The model under review builds one solid part; all positions refer to its coordinate system, in mm. Face numbers are marked on the shaded views. A direction names the side the tool comes from. Round coordinates to 2 decimals unless told otherwise and drop trailing zeros. Return JSON: item names as keys, results as strings.
from build123d import *

# Parameters (mm, degrees)
SKETCH_4_W             = 1
SKETCH_4_H             = 1.2
CUT_EXTRUDE_1_DEPTH    = 50
PATTERN_LINEAR_1_COUNT = 19
PATTERN_LINEAR_1_PITCH = 0.7


with BuildPart() as part:
    # 草图3 → Revolve 915 (revolve)
    with BuildSketch(Plane.XY, mode=Mode.PRIVATE) as revolve_915_sk:
        with BuildLine():
            Line((0, 0), (16.4, 0))
            Line((16.4, 0), (16.4, 2))
            Line((16.4, 2), (3.8, 2))
            Line((3.8, 2), (3.532, 1.732))
            Line((3.532, 1.732), (3.018, 1.732))
            ThreePointArc((3.018, 1.732), (2.581008009, 1.913008009), (2.4, 2.35))
            Line((2.4, 2.35), (2.4, 4))
            Line((2.4, 4), (1.095413109, 3.885863436))
            ThreePointArc((1.095413109, 3.885863436), (0.315267196, 3.501138048), (0, 2.690429799))
            Line((0, 2.690429799), (0, 0))
        make_face()
    revolve(revolve_915_sk.sketch.rotate(Axis((-2.477021524, 0, 0), (1, 0, 0)), 90), axis=Axis((-2.477021524, 0, 0), (1, 0, 0)))

    # 草图4 → 切除-拉伸1 (cut, symmetric)
    with BuildSketch(Plane.XY):
        with Locations((0.5, 0)):
            Rectangle(SKETCH_4_W, SKETCH_4_H)
    extrude(amount=CUT_EXTRUDE_1_DEPTH, both=True, mode=Mode.SUBTRACT)

    # 草图5 → 切除-旋转1 (revolve, cut)
    with BuildSketch(Plane.XY, mode=Mode.PRIVATE) as cut_revolve_1_sk:
        Polygon((16.046208796, 2), (16.746208796, 2), (16.4, 1.3938), align=None)
    cut_revolve_1 = revolve(cut_revolve_1_sk.sketch.rotate(Axis((6.174994867, 0, 0), (-1, 0, 0)), 270), axis=Axis((6.174994867, 0, 0), (-1, 0, 0)), mode=Mode.SUBTRACT)

    # 阵列(线性)1: 切除-旋转1 ×19
    with Locations(*[(-i * PATTERN_LINEAR_1_PITCH, 0, 0) for i in range(1, PATTERN_LINEAR_1_COUNT)]):
        add(cut_revolve_1, mode=Mode.SUBTRACT)


solid = part.part
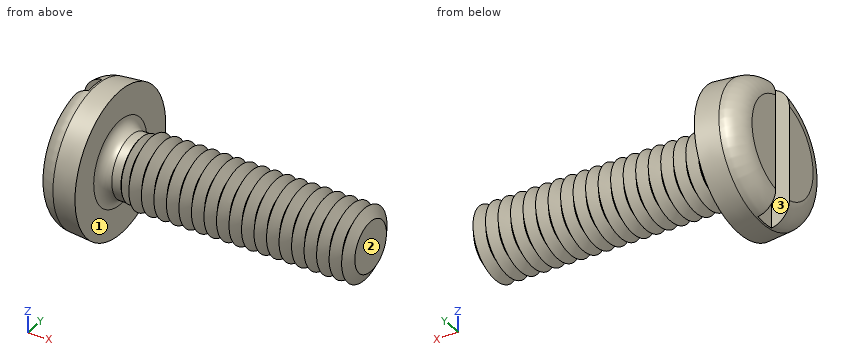
(1) Clearance check with flat-ended pins moving along their axes: pin 1 Ø0.8 at (x, z) = (0.5, 1.5) entering from -Y; pin 2 Ø2 at (x, z) = (10.5, 1.5) entering from +Y; pin 3 Ø3 at (x, y) = (14.5, 2) entering from +Z. State where each tip first meets the part, or that it passes through.
Filled in:
{"pin 1": "stops at y = -3.62", "pin 2": "stops at y = 1.94", "pin 3": "stops at z = 1.93"}
(2) Wall thickness on line 1 (X direction, y = 1.5, z = -1.75); line 2 (X direction, y = 0, z = -0.75); line 3 (Z direction, x = 12.75, y = -1): over which ranges is each line inside the solid? List them lowest first.
Filled in:
{"line 1": "x = 0 to 2.4", "line 2": "x = 1 to 16.4", "line 3": "z = -1.31 to 1.31"}
(3) For the marked faces 1, 2 and 3, list the 3-axis set-ups (+Z, -Z, +X, -X, +Y, -Y) from which the entire face can be reached by the end or side of a thin tool; tool diameter is ignored.
Filled in:
{"face 1": "+X", "face 2": "+Z, -Z, +X, +Y, -Y", "face 3": "+Z, -Z, -X"}
